Source: CAD feature listing. Evaluate the final solid. Frame: model axes, mm. A direction names the side the tool comes from. Give positions to 0.01 mm unless a question says otherwise; leave off trailing zeros. Order: outer loops, then holes, each group sorted by start corner. A loop starts at its lowest first (then second) coordinate and runs counter-clockwise, first axis right, second up. Notation, with made-up numbers: M 40,13 L 61,13 A25 ccw 61,25 Z; hole C 76.25,-18.5 d1. An arc over 180 degrees is marked long. One line per question, with ' | ' between items. Start each with the question number.
from build123d import *

# Parameters (mm, degrees)
SKETCH033_R             = 1.65
SKETCH033_R_2           = 3.7
PAD001_DEPTH            = 3
CHAMFER001_SIZE         = 2
CHAMFER002_SIZE         = 1.4
SKETCH035_R             = 1.5
POCKET009_DEPTH         = 1.5
BODY005_PLACEMENT_ANGLE = 340


with BuildPart() as part:
    # Sketch033 → Pad001 (new body)
    with BuildSketch(Plane.XZ):
        with BuildLine():
            Line((-33.806498, 37.4), (33.806497, 37.4))
            ThreePointArc((41.8, 29.722351), (39.348211, 35.169697), (33.806497, 37.4))
            Line((41.8, 29.722351), (42.55, 11.122345))
            ThreePointArc((34.556497, 2.8), (40.326192, 5.258284), (42.55, 11.122345))
            Line((34.556497, 2.8), (-34.556497, 2.8))
            ThreePointArc((-42.55, 11.122345), (-40.326192, 5.258284), (-34.556497, 2.8))
            Line((-42.55, 11.122345), (-41.8, 29.722351))
            ThreePointArc((-33.806498, 37.4), (-39.348211, 35.169697), (-41.8, 29.722351))
        make_face()
        with Locations((-36.75, 32.1)):
            Circle(SKETCH033_R, mode=Mode.SUBTRACT)
        with Locations((36.75, 32.1)):
            Circle(SKETCH033_R, mode=Mode.SUBTRACT)
        with Locations((-38, 8.1)):
            Circle(SKETCH033_R, mode=Mode.SUBTRACT)
        with Locations((38, 8.1)):
            Circle(SKETCH033_R, mode=Mode.SUBTRACT)
        with Locations((25.5, 22.3)):
            Circle(SKETCH033_R_2, mode=Mode.SUBTRACT)
        with BuildLine():
            Line((-11.25, 29.35), (8.75, 29.35))
            ThreePointArc((11, 27.1), (10.34099, 28.69099), (8.75, 29.35))
            Line((11, 27.1), (11, 18.5))
            ThreePointArc((8.75, 16.25), (10.34099, 16.90901), (11, 18.5))
            Line((8.75, 16.25), (-11.25, 16.25))
            ThreePointArc((-13.5, 18.5), (-12.84099, 16.90901), (-11.25, 16.25))
            Line((-13.5, 18.5), (-13.5, 27.1))
            ThreePointArc((-11.25, 29.35), (-12.84099, 28.69099), (-13.5, 27.1))
        make_face(mode=Mode.SUBTRACT)
        with BuildLine():
            Line((-30.35, 25.929165), (-25.65, 25.929165))
            ThreePointArc((-25.65, 14.670835), (-21.9, 20.3), (-25.65, 25.929165))
            Line((-30.35, 14.670835), (-25.65, 14.670835))
            ThreePointArc((-30.35, 25.929165), (-34.1, 20.3), (-30.35, 14.670835))
        make_face(mode=Mode.SUBTRACT)
    extrude(amount=PAD001_DEPTH)

    # Chamfer001
    chamfer001_edges = [part.edges().sort_by_distance(p)[0] for p in [
        (-1.25, -3, 29.35),
    ]]
    chamfer(chamfer001_edges, length=CHAMFER001_SIZE)

    # Chamfer002
    chamfer002_edges = [part.edges().sort_by_distance(p)[0] for p in [
        (-38.4, -3, 32.1),
        (-39.65, -3, 8.1),
        (35.1, -3, 32.1),
        (36.35, -3, 8.1),
    ]]
    chamfer(chamfer002_edges, length=CHAMFER002_SIZE)

    # Sketch035 → Pocket009 (cut)
    with BuildSketch(Plane.XZ):
        with Locations((25.5, 29.3)):
            Circle(SKETCH035_R)
    extrude(amount=POCKET009_DEPTH, mode=Mode.SUBTRACT)


with BuildPart() as part_1:
    # Body005 placement: moved
    add(part.part.moved(Location((0, -38, 0))).rotate(Axis((0, -38, 0), (1, 0, 0)), BODY005_PLACEMENT_ANGLE))


solid = part_1.part
Item 1: Cut plane B-B on z = 23.5. Count the separate pieces of the cut face and the enclosed holes in it, and give its area (3 significant figures).
Item 2: Mould query, pull axis X, two halves, no side actions, for faces 1 (the cylindrical face through (40.263, -37.614, 5.386)), 2 (the flat face through (12.01, -32.07, 22.17)), 3 (the cylindrical face through (-40.39, -37.57, 5.51)), 4 (the flat face through (-1.39, -29.507, 29.222)). Classes: pulls with the +X half, pulls with the -X half, needs draft (parallel to the pull), parting line crosses it, or undercut.
Item 3: Pin query (flat end, axial travel): pin 1 Ø1 at (x, z) = (-29, 14) entering from +Y; pin 2 Ø2 at (x, z) = (16, 9.5) entering from -Y; pin 3 Ø2 at (x, y) = (20, -27) entering from +Z; pin 4 Ø1 at (y, z) = (-35.5, 21) entering from -X. Return the tip coordinate at first contact, or that it passes through.
Item 4: Reachability of faces 5 (the flat face through (11, -30.6, 21.7)), 6 (the cylindrical face through (-12.82, -28.64, 27.15)), 7 (the flat face through (25.48, -29.38, 28.07)) from +Z, -Z, +X, -X, +Y, -Y: full face, straight path, thin tool, end or side. Return the list, or none.
Item 5: Cut plane C-C on x = -19. Return the cut outline in (y, z), and give its area (3 significant figures).
Item 6: Cut plane A-A on x = -4. Return the cut outline in (y, z).
Item 7: Line query: line 1 (X direction, y = -29.25, z = 31.5); line 2 (X direction, y = -37.75, z = 8); line 3 (Y direction, x = 34, z = 19.5). Output: solid intervals per line, ascending.
Results are:
1) separate pieces: 4 | enclosed holes: 0 | area: 138 mm2
2) face 1: pulls with the +X half | face 2: undercut | face 3: pulls with the -X half | face 4: undercut
3) pin 1: stops at y = -32.98 | pin 2: stops at y = -38.1 | pin 3: stops at z = 36.16 | pin 4: passes through
4) face 5: +Y, -Y | face 6: -Z, -Y | face 7: none
5) outline: M -39.86,3.66 L -37.04,2.63 L -25.21,35.14 L -28.03,36.17 Z | area: 104 mm2
6) outline: M -39.86,3.66 L -37.04,2.63 L -32.44,15.27 L -33.38,15.61 L -35.95,14.42 Z; M -30.1,30.49 L -28.9,27.92 L -27.96,27.58 L -25.21,35.14 L -28.03,36.17 Z
7) line 1: x = -41.14 to -39.3, -34.2 to 34.2, 39.3 to 41.14 | line 2: x = -41.89 to -40.5, -35.5 to 35.5, 40.5 to 41.89 | line 3: y = -34.1 to -30.9
